from build123d import *

# Parameters (mm, degrees)
F2_DEPTH = 2.8
F4_DEPTH = 1.7
F6_DEPTH = 12.5


# Not quite as in the source:
# - a feature of the source that left no trace in its solid (it failed there, or was rolled back) is left out


with BuildPart() as f2:
    # F1 (on Top) → F2 (new body)
    with BuildSketch(Plane.XY):
        with BuildLine():
            Line((-5.1537473182, 3.6727124144), (-5.7416372565, -3.0469003289))
            ThreePointArc((-5.7416372565, -3.0469003289), (0, -6.5), (5.7416372565, -3.0469003289))
            Line((5.7416372565, -3.0469003289), (5.1537473182, 3.6727124144))
            Line((5.1537473182, 3.6727124144), (3.4859795486, 4.7765922388))
            Line((3.4859795486, 4.7765922388), (2.7272692442, 2.9260899627))
            ThreePointArc((2.7272692442, 2.9260899627), (0, -4), (-2.7272692442, 2.9260899627))
            Line((-2.7272692442, 2.9260899627), (-3.4859795486, 4.7765922388))
            Line((-3.4859795486, 4.7765922388), (-5.1537473182, 3.6727124144))
        make_face()
    extrude(amount=F2_DEPTH)

    # F3 (on face) → F4 (join)
    with BuildSketch(Plane.XY.offset(2.8)):
        with BuildLine():
            Line((-4.6721311475, -3.2651478589), (-5.3278688525, -3.723414225))
            ThreePointArc((-5.3278688525, -3.723414225), (0, -6.5), (5.3278688525, -3.723414225))
            Line((5.3278688525, -3.723414225), (4.6721311475, -3.2651478589))
            ThreePointArc((4.6721311475, -3.2651478589), (0, -5.7), (-4.6721311475, -3.2651478589))
        make_face()
    extrude(amount=F4_DEPTH)

    # F5 (on Right) → F6 (cut, symmetric)
    with BuildSketch(Plane.YZ):
        Polygon((6.7765922388, 2.8), (2.9260899627, 2.8), (6.7765922388, 0.5769114744), align=None)
    extrude(amount=F6_DEPTH, both=True, mode=Mode.SUBTRACT)


solid = f2.part
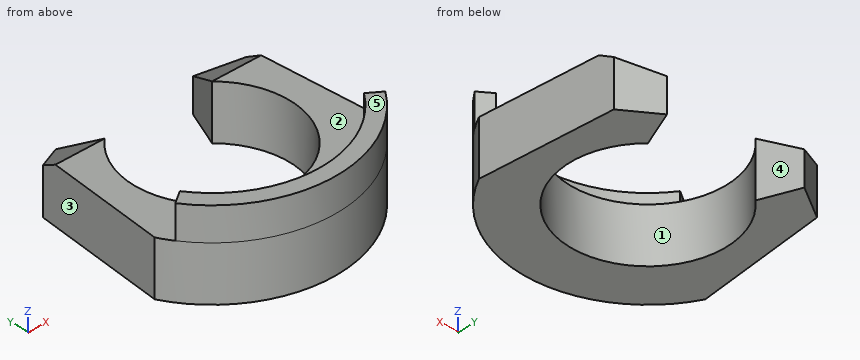
Geometry: final body of the model. Coordinates: model frame, mm. Face numbers are marked on the shaded views. A direction names the side the tool comes from. Give positions to 0.01 mm unless a question says otherwise; leave off trailing zeros. Loops run counter-clockwise (first coordinate to the right, second up) from the corner with the lowest first, then second, coordinate; pieces in that order, holes last. Notation, with made-up numbers: M 44,22.25 L 82,22.25 A20 cw 82,56.25 Z; hole C -39,-19.75 d10. An arc over 180 degrees is marked long. Put each result on its own line as item: value.
1) Mould query, pull axis Y, two halves, no side actions, for the marked faces 1, 2 and 3. Classes: released by +Y, released by -Y, zero draft, split by the parting line, or undercut.
Computed values:
face 1: undercut
face 2: zero draft
face 3: released by +Y
2) Cut plane D-D, the plane x = 3.25. Return the cut outline in (y, z).
Computed values:
outline: M -5.63,0 L -2.33,0 L -2.33,2.8 L -4.68,2.8 L -4.68,4.5 L -5.63,4.5 Z; M 2.33,0 L 4.2,0 L 4.2,2.06 L 2.93,2.8 L 2.33,2.8 Z
3) First-contact query: P1, Ø1.5, axis at y = 3, z = 3, coming from the -X side; P2, Ø1.5, axis at y = -4, z = 4, coming from the +X side; P3, Ø1, axis at y = -1.5, z = 1.5, coming from the +X side. Flat tips, straight axial feed; report the tip coordinate or a pass-through.
Computed values:
P1: stops at x = -5.28
P2: stops at x = 5.33
P3: stops at x = 5.65
4) Cut plane B-B, the plane z = 0.95. Return the cut outline in (x, y), plus the area to 3 significant figures.
Computed values:
outline: M -5.74,-3.05 A6.5 ccw 5.74,-3.05 L 5.15,3.67 L 3.49,4.78 L 2.73,2.93 A4 cw long -2.73,2.93 L -3.49,4.78 L -5.15,3.67 Z
area: 53.3 mm^2
5) Cut plane A-A, the plane y = 1.5. Return the cut outline in (x, z).
Computed values:
outline: M -5.34,0 L -3.71,0 L -3.71,2.8 L -5.34,2.8 Z; M 3.71,0 L 5.34,0 L 5.34,2.8 L 3.71,2.8 Z
6) Material intervals for L1, parallel to Z at x = 5.25, y = -1; L2, parallel to X at y = 0, z = 1.95; L3, parallel to X at y = 2.5, z = 0.75, sorted ascending. Write a range as from..to.
Computed values:
L1: z = 0..2.8
L2: x = -5.48..-4, 4..5.48
L3: x = -5.26..-3.12, 3.12..5.26
7) Cut plane C-C, the plane x = 0. Return the cut outline in (y, z), plus the area to 3 significant figures.
Computed values:
outline: M -6.5,0 L -4,0 L -4,2.8 L -5.7,2.8 L -5.7,4.5 L -6.5,4.5 Z
area: 8.36 mm^2
8) Reachability of the marked faces 4 and 5 from +Z, -Z, +X, -X, +Y, -Y: full face, straight path, thin tool, end or side. Return the list, or none.
Computed values:
face 4: +Z, -Z, +Y
face 5: +Z, +X, -X, +Y, -Y
